Can you work these out from the model? Positions are in its coordinate system, mm. A direction names the side the tool comes from. Give positions to 0.01 mm unless a question says otherwise; leave off trailing zeros. Order: outer loops, then holes, each group sorted by start corner. A loop starts at its lowest first (then second) coordinate and runs counter-clockwise, first axis right, second up. Notation, with made-up numbers: M 42.5,17 L 99.5,17 A35 cw 99.5,51 Z; hole C 78.5,57.25 d9. An arc over 180 degrees is marked long. Use one line per item in the form item = value. Start each with the question number.
1. I want a section at C-C, the plane y = -75.5. List the corners of the cut face in (x, z) for me, and give its area (3 significant figures).
2. We'd pull the mould along Y, two halves only. Please class faces 1 (the face through (599, 1000, 49)), 2 (the face through (537.675, -164.05, -86.445)), 3 (the face through (700, -951, 51)): +Y half, -Y half, draft (parallel to the pull), parting line (faces both ways), or undercut.
3. I want a section at B-B, the plane z = -429.5. List the corners of the cut face in (x, y) for me.
4. I want a section at D-D, the plane z = -34. List the corners of the cut face in (x, y) for me.
5. I need wall thicknesses on L1, parallel to Z at x = -184, y = 304.5; L2, parallel to X at y = 734.5, z = 82.5; L3, parallel to Y at x = -532, z = -548. Which ranges of each line are inside material? Lowest first, please.
6. I want a section at A-A, the plane y = 814. List the corners of the cut face in (x, z) for me, and give its area (3 significant figures).
7. For faces 4 (the face through (538, 160, -92)), 5 (the face through (599, -670, 100)), 6 (the face through (674.65, 997.69, 65.02)), 7 (the face through (650, 988, 10)), which set-ups out of +Z, -Z, +X, -X, +Y, -Y let a thin tool reach every point of the face, with its end or its side?
```python
from build123d import *

# Parameters (mm, degrees)
F0_W      = 100
F0_H      = 2000
F1_DEPTH  = 100
F2_W      = 1300
F2_H      = 50
F3_DEPTH  = 25
F4_R      = 50
F5_DEPTH  = 50
F6_R      = 50
F7_DEPTH  = 50
F9_DEPTH  = 25
F11_DEPTH = 25
F12_R     = 30


with BuildPart() as f1:
    # F0 (on Top) → F1 (new body)
    with BuildSketch(Plane.XY):
        with Locations((600, 0)):
            Rectangle(F0_W, F0_H)
        with Locations((-600, 0)):
            Rectangle(F0_W, F0_H)
    extrude(amount=F1_DEPTH)

    # F2 (on face) → F3 (join)
    with BuildSketch(Plane.XY.offset(100)):
        with Locations((0, -325)):
            Rectangle(F2_W, F2_H)
        with Locations((0, 325)):
            Rectangle(F2_W, F2_H)
    extrude(amount=F3_DEPTH)

    # F4 (on face) → F5 (join)
    with BuildSketch(Plane(origin=(-650, 0, 0), x_dir=(0, -1, 0), z_dir=(-1, 0, 0))):
        with Locations((-950, 50)):
            Circle(F4_R)
        with Locations((950, 50)):
            Circle(F4_R)
    extrude(amount=F5_DEPTH)

    # F6 (on face) → F7 (join)
    with BuildSketch(Plane.YZ.offset(650)):
        with Locations((-950, 50)):
            Circle(F6_R)
        with Locations((950, 50)):
            Circle(F6_R)
    extrude(amount=F7_DEPTH)

    # F8 (on face) → F9 (join)
    with BuildSketch(Plane.YZ.offset(-550)):
        Polygon((-300, 100), (-350, 100), (-25, -345.714286), (-25, -745.714286), (25, -745.714286), (25, -345.714286), (350, 100), (300, 100), (0, -311.428571), align=None)
    extrude(amount=F9_DEPTH)

    # F10 (on face) → F11 (join)
    with BuildSketch(Plane(origin=(550, 0, 0), x_dir=(0, -1, 0), z_dir=(-1, 0, 0))):
        Polygon((25, -345.714286), (350, 100), (300, 100), (0, -311.428571), (-300, 100), (-350, 100), (-25, -345.714286), (-25, -745.714286), (25, -745.714286), align=None)
    extrude(amount=F11_DEPTH)

    # F12
    f12_edges = [f1.edges().sort_by_distance(p)[0] for p in [
        (-537.5, 0, -311.428571),
        (537.5, 0, -311.428571),
    ]]
    fillet(f12_edges, radius=F12_R)


solid = f1.part
```
Check result:
q1.outline = M -650,0 L -550,0 L -550,100 L -650,100 Z; M -550,-276.46 L -525,-276.46 L -525,-207.89 L -550,-207.89 Z; M 525,-276.46 L 550,-276.46 L 550,-207.89 L 525,-207.89 Z; M 550,0 L 650,0 L 650,100 L 550,100 Z
q1.area = 23,400 mm2
q2.face_1 = +Y half
q2.face_2 = undercut
q2.face_3 = draft
q3.outline = M -550,-25 L -525,-25 L -525,25 L -550,25 Z; M 525,-25 L 550,-25 L 550,25 L 525,25 Z
q4.outline = M -550,-252.29 L -525,-252.29 L -525,-202.29 L -550,-202.29 Z; M -550,202.29 L -525,202.29 L -525,252.29 L -550,252.29 Z; M 525,-252.29 L 550,-252.29 L 550,-202.29 L 525,-202.29 Z; M 525,202.29 L 550,202.29 L 550,252.29 L 525,252.29 Z
q5.L1 = 100 to 125
q5.L2 = -650 to -550, 550 to 650
q5.L3 = -25 to 25
q6.outline = M -650,0 L -550,0 L -550,100 L -650,100 Z; M 550,0 L 650,0 L 650,100 L 550,100 Z
q6.area = 20,000 mm2
q7.face_4 = +Z
q7.face_5 = +Z, +X, -X, -Y
q7.face_6 = +X
q7.face_7 = -Z, +X, +Y
